Can you work these out from the model? Positions are in its coordinate system, mm. Coordinates: 2 decimals unless noted, no trailing zeros. Order: outer loops, then holes, each group sorted by start corner. A loop starts at its lowest first (then second) coordinate and runs counter-clockwise, first axis right, second up. Notation, with made-up numbers: (-19, 20) -> (-14, 20) arc R30 cw to (-14, 59) -> close; hole circle Ø2 at (-5.5, 6). An arc over 180 degrees is marked (long way). Answer as CSV lines item,"result".
from build123d import *

# Parameters (mm, degrees)
SKETCH2_R               = 1.25
BOSS_EXTRUDE1_DEPTH     = 2
CUT_EXTRUDE1_DEPTH      = 12.357816692
CUT_EXTRUDE1_DEPTH_BACK = 12.357816692
SKETCH3_W               = 5
SKETCH3_H               = 1
FILLET1_R               = 2
BOSS_EXTRUDE2_START     = 20
BOSS_EXTRUDE2_DEPTH     = 20
SKETCH6_R               = 1.5
CUT_EXTRUDE2_DEPTH      = 25.677925359


with BuildPart() as part:
    # Sketch2 → Boss-Extrude1 (new body)
    with BuildSketch(Plane(origin=(0, 0, 0), x_dir=(1, 0, 0), z_dir=(0, 1, 0))):
        with BuildLine():
            Line((-8.333333333, -2.357022604), (-1.666666667, -4.714045208))
            ThreePointArc((-1.666666667, -4.714045208), (0, -5), (1.666666667, -4.714045208))
            Line((1.666666667, -4.714045208), (8.333333333, -2.357022604))
            ThreePointArc((8.333333333, -2.357022604), (10, 0), (8.333333333, 2.357022604))
            Line((8.333333333, 2.357022604), (1.666666667, 4.714045208))
            ThreePointArc((1.666666667, 4.714045208), (0, 5), (-1.666666667, 4.714045208))
            Line((-1.666666667, 4.714045208), (-8.333333333, 2.357022604))
            ThreePointArc((-8.333333333, 2.357022604), (-10, 0), (-8.333333333, -2.357022604))
        make_face()
        with Locations(Location((-7.5, 0, 0), (0, 0, 270))):
            Circle(SKETCH2_R, mode=Mode.SUBTRACT)
        with Locations(Location((7.5, 0, 0), (0, 0, 270))):
            Circle(SKETCH2_R, mode=Mode.SUBTRACT)
    extrude(amount=BOSS_EXTRUDE1_DEPTH)

    # Sketch3 → Cut-Extrude1 (cut, two sides: drawn at the far end of the back side and taken through both)
    with BuildSketch(Plane.XY.offset(-CUT_EXTRUDE1_DEPTH_BACK)):
        with Locations((-7.5, 0.5)):
            Rectangle(SKETCH3_W, SKETCH3_H)
        with Locations((7.5, 0.5)):
            Rectangle(SKETCH3_W, SKETCH3_H)
    extrude(amount=CUT_EXTRUDE1_DEPTH + CUT_EXTRUDE1_DEPTH_BACK, mode=Mode.SUBTRACT)

    # Fillet1
    fillet1_edges = [part.edges().sort_by_distance(p)[0] for p in [
        (-5, 0.5, -3.535533906),
        (5, 0.5, -3.535533906),
        (-5, 0.5, 3.535533906),
        (5, 0.5, 3.535533906),
    ]]
    fillet(fillet1_edges, radius=FILLET1_R)

    # Sketch5 → Boss-Extrude2 (add)
    with BuildSketch(Plane.XZ.offset(BOSS_EXTRUDE2_START)):
        with BuildLine():
            Line((5, -2.121320344), (5, 2.121320344))
            ThreePointArc((5, 2.121320344), (4.632993162, 3.276020882), (3.666666667, 4.006938427))
            Line((3.666666667, 4.006938427), (1.666666667, 4.714045208))
            ThreePointArc((1.666666667, 4.714045208), (0, 5), (-1.666666667, 4.714045208))
            Line((-1.666666667, 4.714045208), (-3.666666667, 4.006938427))
            ThreePointArc((-3.666666667, 4.006938427), (-4.632993162, 3.276020882), (-5, 2.121320344))
            Line((-5, 2.121320344), (-5, -2.121320344))
            ThreePointArc((-5, -2.121320344), (-4.632993162, -3.276020882), (-3.666666667, -4.006938427))
            Line((-3.666666667, -4.006938427), (-1.666666667, -4.714045208))
            ThreePointArc((-1.666666667, -4.714045208), (0, -5), (1.666666667, -4.714045208))
            Line((1.666666667, -4.714045208), (3.666666667, -4.006938427))
            ThreePointArc((3.666666667, -4.006938427), (4.632993162, -3.276020882), (5, -2.121320344))
        make_face()
    extrude(amount=-BOSS_EXTRUDE2_DEPTH)

    # Sketch6 → Cut-Extrude2 (cut, through all)
    with BuildSketch(Plane.XZ.offset(20)):
        with Locations(Location((-2.5, 0, 0), (0, 0, 270))):
            Circle(SKETCH6_R)
        with Locations(Location((2.5, 0, 0), (0, 0, 270))):
            Circle(SKETCH6_R)
    extrude(amount=-CUT_EXTRUDE2_DEPTH, mode=Mode.SUBTRACT)


solid = part.part
Q1. Imagine slicing it at A-A (y = -9.25). List the corners of the cut face in (x, z) for me.
Solution:
outline,"(-5, -2.12) arc R2 ccw to (-3.67, -4.01) -> (-1.67, -4.71) arc R5 ccw to (1.67, -4.71) -> (3.67, -4.01) arc R2 ccw to (5, -2.12) -> (5, 2.12) arc R2 ccw to (3.67, 4.01) -> (1.67, 4.71) arc R5 ccw to (-1.67, 4.71) -> (-3.67, 4.01) arc R2 ccw to (-5, 2.12) -> close; hole circle Ø3 at (-2.5, 0); hole circle Ø3 at (2.5, 0)"
Q2. For P1, Ø2.5, axis at x = 2.5, z = 0, coming from the -Y side; P2, Ø4.5, axis at y = -9, z = 0, coming from the +X side; P3, Ø3.5, axis at x = -2.5, z = 0, coming from the -Y side; P4, Ø2, axis at y = -8, z = 2.5, coming from the -X side, each with a flat end and sliding along its axis, tell me the tip position at first contact or that it passes through.
Solution:
P1,"through"
P2,"x = 5"
P3,"y = -20"
P4,"x = -5"
Q3. We'd pull the mould along X, two halves only. Please class faces 1 (the cylindrical face through (6.28, 1.49, -0.27)), 2 (the flat face through (5, -10, 0)), 3 (the flat face through (-5, -10, 0)): pulls with the +X half, pulls with the -X half, needs draft (parallel to the pull), parting line crosses it, or undercut.
Solution:
face 1,"undercut"
face 2,"pulls with the +X half"
face 3,"pulls with the -X half"
Q4. Imagine slicing it at B-B (x = 2.5). List the corners of the cut face in (y, z) for me, and give its area (3 significant figures).
Solution:
outline,"(-20, -4.42) -> (2, -4.42) -> (2, -1.5) -> (-20, -1.5) -> close; (-20, 1.5) -> (2, 1.5) -> (2, 4.42) -> (-20, 4.42) -> close"
area,"128 mm2"
Q5. Imagine slicing it at C-C (z = -3.5). List the corners of the cut face in (x, y) for me.
Solution:
outline,"(-5.1, 1) -> (-4.45, 1) -> (-4.45, -20) -> (4.45, -20) -> (4.45, 1) -> (5.1, 1) -> (5.1, 2) -> (-5.1, 2) -> close"
Q6. Imagine slicing it at D-D (x = -7.5). List the corners of the cut face in (y, z) for me.
Solution:
outline,"(1, -2.65) -> (2, -2.65) -> (2, -1.25) -> (1, -1.25) -> close; (1, 1.25) -> (2, 1.25) -> (2, 2.65) -> (1, 2.65) -> close"
Q7. If I drill on line 1 (X direction, y = -11.25, z = 0); line 2 (X direction, y = 1.5, z = 0); line 3 (X direction, y = -1.5, z = 0.5), over which ranges is the centre line in solid material (lowest first)?
Solution:
line 1,"-5 to -4, -1 to 1, 4 to 5"
line 2,"-10 to -8.75, -6.25 to -4, -1 to 1, 4 to 6.25, 8.75 to 10"
line 3,"-5 to -3.91, -1.09 to 1.09, 3.91 to 5"
